```python
from build123d import *

# Parameters (mm, degrees)
CROQUIS1_R              = 37.5
SALIENTE_EXTRUIR1_DEPTH = 2.5
CROQUIS3_W              = 2
CROQUIS3_H              = 4
CROQUIS5_R              = 35
CROQUIS5_R_2            = 34
SALIENTE_EXTRUIR2_DEPTH = 2.5


with BuildPart() as part:
    # Croquis1 → Saliente-Extruir1 (new body)
    with BuildSketch(Plane(origin=(0, 0, 0), x_dir=(1, 0, 0), z_dir=(0, 1, 0))):
        with Locations((13.541348433, 6.626768313)):
            Circle(CROQUIS1_R)
        with BuildLine():
            Line((13.541348433, 41.626768313), (13.541348433, 11.626768313))
            ThreePointArc((13.541348433, 11.626768313), (17.076882339, 10.162302219), (18.541348433, 6.626768313))
            Line((18.541348433, 6.626768313), (48.541348433, 6.626768313))
            ThreePointArc((48.541348433, 6.626768313), (38.290085775, 31.375505654), (13.541348433, 41.626768313))
        make_face(mode=Mode.SUBTRACT)
        with BuildLine():
            Line((8.541348433, 6.626768313), (-21.458651567, 6.626768313))
            ThreePointArc((-21.458651567, 6.626768313), (-11.207388908, -18.121969029), (13.541348433, -28.373231687))
            Line((13.541348433, -28.373231687), (13.541348433, 1.626768313))
            ThreePointArc((13.541348433, 1.626768313), (10.005814527, 3.091234407), (8.541348433, 6.626768313))
        make_face(mode=Mode.SUBTRACT)
    extrude(amount=SALIENTE_EXTRUIR1_DEPTH)

    # Barrer1: sweep along a path in Croquis4
    with BuildLine(Plane(origin=(0, 0, 0), x_dir=(-1, 0, 0), z_dir=(0, -1, 0))) as barrer1_path:
        CenterArc((-13.541348433, 6.626768313), 36.25, 0, 360)
    # Croquis3 → Barrer1 (sweep)
    with BuildSketch(Plane.XY.offset(-6.626768313)):
        with Locations((-22.208651567, -1.9)):
            Rectangle(CROQUIS3_W, CROQUIS3_H)
    sweep(path=barrer1_path.line)

    # Croquis5 → Saliente-Extruir2 (add)
    with BuildSketch(Plane.XZ):
        with Locations((13.541348433, -6.626768313)):
            Circle(CROQUIS5_R)
        with Locations((13.541348433, -6.626768313)):
            Circle(CROQUIS5_R_2, mode=Mode.SUBTRACT)
    extrude(amount=-SALIENTE_EXTRUIR2_DEPTH)


solid = part.part
```
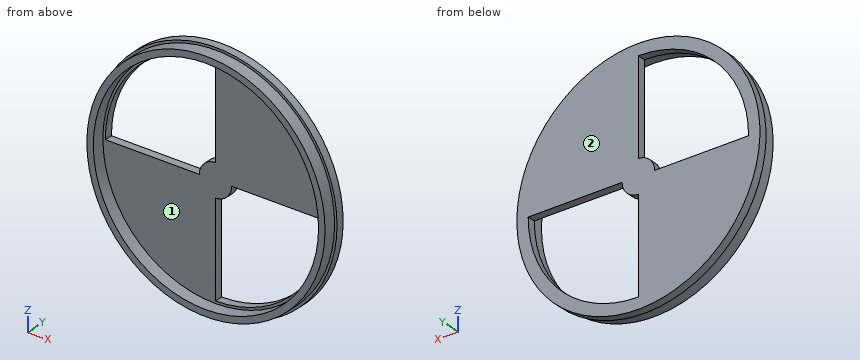
Design review of the part built by this model. Coordinates are the model's own, in mm. Face numbers are marked on the shaded views. Give positions to 0.01 mm unless a question says otherwise; leave off trailing zeros. Loops run counter-clockwise (first coordinate to the right, second up) from the corner with the lowest first, then second, coordinate; pieces in that order, holes last. Notation, with made-up numbers: (53.25, 79) -> (72.25, 79) arc R12 cw to (72.25, 85) -> close; hole circle Ø4 at (71.25, 10.5). An arc over 180 degrees is marked (long way). Write each question's results on one line, items separated by ' | '.
Q1. For pin 1 Ø3 at (y, z) = (-2.5, 14.5) entering from -X; pin 2 Ø10 at (x, z) = (4.5, -9.5) entering from -Y; pin 3 Ø0.8 at (y, z) = (1, -26.5) entering from +X, all flat-tipped, find the tip position at first contact; note any pin that passes through.
Reply:
pin 1: stops at x = -17.53 | pin 2: stops at y = 0 | pin 3: stops at x = 45.59
Q2. Take a section at A-A, the plane y = 1.25. Write out the cut boundary in (x, z), plus the area to 3 significant figures.
Reply:
outline: circle Ø75 at (13.54, -6.63); hole (-20.46, -6.63) -> (8.54, -6.63) arc R5 cw to (13.54, -1.63) -> (13.54, 27.37) arc R34 ccw to start; hole (13.54, -40.63) arc R34 ccw to (47.54, -6.63) -> (18.54, -6.63) arc R5 cw to (13.54, -11.63) -> close | area: 2,640 mm²
Q3. Wall thickness on L1, parallel to Z at x = 14, y = -0.25; L2, parallel to Y at x = 9, z = -5; L3, parallel to X at y = -1.5, z = 16: over which ranges is each line inside the solid? List them lowest first.
Reply:
L1: z = -43.37 to -41.37, 28.12 to 30.12 | L2: y = 0 to 2.5 | L3: x = -15.42 to -12.83, 39.92 to 42.5
Q4. The part is to be moulded in two halves that separate along X. For the marked faces 1 and 2, say which applies: +X half, -X half, draft (parallel to the pull), parting line (faces both ways), or undercut.
Reply:
face 1: undercut | face 2: draft
